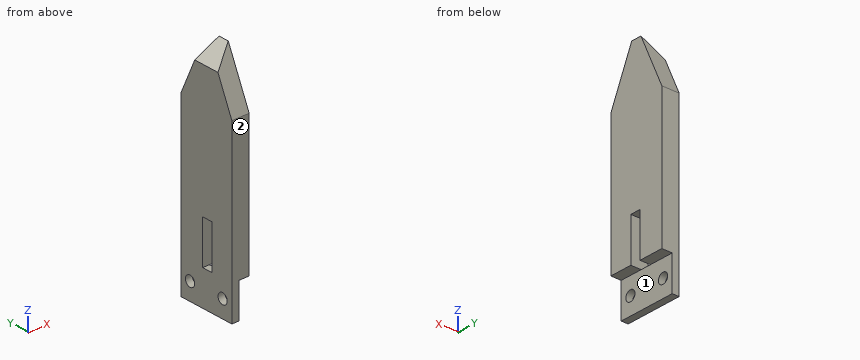
Autodesk Inventor part; units mm, degrees
ref_plane "YZ Plane" through (0, 0, 0) normal (1, 0, 0) x (0, 1, 0)
ref_plane "XZ Plane" through (0, 0, 0) normal (0, 1, 0) x (-1, 0, 0)
ref_plane "XY Plane" through (0, 0, 0) normal (0, 0, 1) x (1, 0, 0)
sketch "スケッチ1" plane through (0, 0, 0) normal (1, 0, 0) x (0, 1, 0)
  line L0 (9.2985, 24.3383) -> (-7.3015, 24.3383)
  line L1 (-7.3015, 24.3383) -> (-7.3015, -40.6617)
  line L2 (-7.3015, -40.6617) -> (9.2985, -40.6617)
  line L3 (9.2985, -40.6617) -> (9.2985, 24.3383)
  line L4 (-7.3015, -40.6617) -> (9.2985, -40.6617)
  line L5 (9.2985, -40.6617) -> (9.2985, -30.6617)
  line L6 (9.2985, -30.6617) -> (-7.3015, -30.6617)
  line L7 (-7.3015, -30.6617) -> (-7.3015, -40.6617)
  circle A0 centre (6.2985, -35.6617) radius 1.5
  circle A1 centre (-4.3015, -35.6617) radius 1.5
  line L8 (2.4985, 24.3383) -> (9.2985, 9.3383)
  line L9 (-0.5015, 24.3383) -> (-7.3015, 9.3383)
  point P0 (0, 0)
  dimension "d0" = 16.6
  dimension "d1" = 10
  dimension "d2" = 3
  dimension "d3" = 3
  dimension "d4" = 5
  dimension "d5" = 5
  dimension "d6" = 3
  dimension "d7" = 3
  dimension "d8" = 3
  dimension "d9" = 15
  dimension "d10" = 15
  dimension "d11" = 6.8
  dimension "d12" = 6.8
  dimension "d13" = 40
extrude "押し出し1" add sketch "スケッチ1" against normal blind 2 contours L8 L3 L6 L1 L9 L0 | L3 L2 L1 L6
extrude "押し出し2" add sketch "スケッチ1" along normal blind 3 contours L8 L3 L6 L1 L9 L0
sketch "スケッチ2" plane through (-2, 9.2985, -40.6617) normal (0, 1, 0) x (1, 0, 0)
  line L0 (5, -50) -> (5, -10)
  line L1 (0, 0) -> (0, -50)
  line L2 (5, -10) -> (0, -10)
  line L3 (0, -10) -> (0, -10.7373)
  line L4 (0, -10.7373) -> (5, -10.7373)
  line L5 (5, -10.7373) -> (5, -10)
  line L6 (5, -22.5) -> (0, -22.5)
  line L7 (0, -22.5) -> (0, -27.5)
  line L8 (0, -27.5) -> (5, -27.5)
  line L9 (5, -27.5) -> (5, -22.5)
  point P0 (2, -40.6617)
  dimension "d18" = 12.5
  dimension "d19" = 5
extrude "押し出し3" add sketch "スケッチ2" along normal blind 3 contours L8 L1 L6 L0
chamfer "面取り1" distance 5 angle 45 1 edges at (-2, 0.9985, 24.3383)
sketch "スケッチ3" plane through (-2, 9.2985, -40.6617) normal (0, 1, 0) x (1, 0, 0)
  line L0 (5, -50) -> (5, -10)
  line L1 (0, -22.5) -> (5, -22.5)
  line L2 (5, -22.5) -> (5, -10)
  line L3 (5, -10) -> (0, -10)
  line L4 (0, -10) -> (0, -22.5)
  point P0 (2, -40.6617)
extrude "押し出し4" cut sketch "スケッチ3" against normal blind 10.1
sketch "スケッチ4" plane through (3, 12.2985, -18.1617) normal (0, 0, -1) x (-1, 0, 0)
  line L0 (0, 0) -> (5, 0)
  line L1 (5, 0) -> (0, 0)
  line L2 (0, 0) -> (0, -10.1)
  line L3 (0, -10.1) -> (5, -10.1)
  line L4 (5, -10.1) -> (5, 0)
  line L5 (0, -13.1) -> (5, -13.1)
  point P0 (3, -12.2985)
  dimension "d27" = 3
extrude "押し出し5" add sketch "スケッチ4" along normal blind 12.5
sketch "スケッチ5" plane through (-2, 12.2985, -40.6617) normal (0, 1, 0) x (1, 0, 0)
  line L0 (5, -10) -> (5, -22.5)
  line L1 (0, -27.5) -> (0, -10)
  line L2 (5, -10) -> (0, -10)
  line L3 (0, -10) -> (0, -27.5)
  line L4 (0, -27.5) -> (5, -27.5)
  line L5 (5, -27.5) -> (5, -10)
  point P0 (2, -40.6617)
extrude "押し出し6" cut sketch "スケッチ5" against normal blind 3
properties part number "armmodulepart1"
CAD build for the part. Positions are in the model's coordinates, mm. Face numbers are marked on the shaded views. A direction names the side the tool comes from. Round coordinates to 2 decimals unless told otherwise and drop trailing zeros. Loops run counter-clockwise (first coordinate to the right, second up) from the corner with the lowest first, then second, coordinate; pieces in that order, holes last. Notation, with made-up numbers: M -10,86 L -1,86 A7 cw -1,92 Z; hole C 30,22 d4. An arc over 180 degrees is marked long. Use a Markdown table: item, result. Add a question column.
(1) Cut at C-C (x = -0.7). Give the cut face in (y, z), and give its area (3 significant figures).
(2) Cut at B-B (y = -4.5). Give the cut face in (x, z), and give its area (3 significant figures).
(3) Cut at D-D (z = -32). Give the cut face in (x, y), and give its area (3 significant figures).
(4) Cut at A-A (z = -24.5). Give the cut face in (x, y), and give its area (3 significant figures).
(5) Which spindle directions (+Z, -Z, +X, -X, +Y, -Y) get a long thin tool onto all of the face, cutting with end or side? Do the marked faces 1 and 2. Say none if no direction does.
(6) Flat gauge pins, fed straight in: pin 1 (2 mm diameter, centred on x = 1, z = 17.5, fed in from +Y); pin 2 (1.6 mm diameter, centred on x = -1, y = 0.5, fed in from +Z); pin 3 (1.5 mm diameter, centred on x = 0.5, y = 6.5, fed in from -Z); pin 4 (2.5 mm diameter, centred on y = -4.3, z = -35.66, fed in from +X). Where does each tip first touch, or does it go through?
(7) Drill centre lines: line 1 (Y direction, x = -1.35, z = -35.5); line 2 (Y direction, x = 0.5, z = -21.5); line 3 (Z direction, x = -1.7, y = 1). Where is each one in solid material? Low to high.
Geometry says:
| question | item | result |
|---|---|---|
| 1 | outline | M -7.3,-40.66 L 9.3,-40.66 L 9.3,9.34 L 4.18,20.64 L -2.18,20.64 L -7.3,9.34 Z; hole C -4.3,-35.66 d3; hole M -0.8,-30.66 L 2.2,-30.66 L 2.2,-18.16 L -0.8,-18.16 Z; hole C 6.3,-35.66 d3 |
| 1 | area | 908 mm² |
| 2 | outline | M -2,-40.66 L 0,-40.66 L 0,-37.15 L -2,-37.15 Z; M -2,-34.17 L 0,-34.17 L 0,-30.66 L 3,-30.66 L 3,15.52 L -2,15.52 Z |
| 2 | area | 245 mm² |
| 3 | outline | M -2,-7.3 L 0,-7.3 L 0,9.3 L -2,9.3 Z |
| 3 | area | 33.2 mm² |
| 4 | outline | M -2,-7.3 L 3,-7.3 L 3,-0.8 L -2,-0.8 Z; M -2,2.2 L 3,2.2 L 3,9.3 L -2,9.3 Z |
| 4 | area | 68.0 mm² |
| 5 | face 1 | -Z, +X, +Y, -Y |
| 5 | face 2 | +Z, -Z, +X, -X, -Y |
| 6 | pin 1 | stops at y = 6.05 |
| 6 | pin 2 | stops at z = 21.14 |
| 6 | pin 3 | stops at z = -40.66 |
| 6 | pin 4 | passes through |
| 7 | line 1 | y = -7.3 to -5.79, -2.81 to 4.81, 7.79 to 9.3 |
| 7 | line 2 | y = -7.3 to -0.8, 2.2 to 9.3 |
| 7 | line 3 | z = -40.66 to -30.66, -18.16 to 19.64 |
